Here's how the part is built. I have some questions about the finished solid (model axes, mm). Face numbers are marked on the shaded views. A direction names the side the tool comes from. Coordinates: 2 decimals unless noted, no trailing zeros. Write each loop counter-clockwise with the first axis right and the second up, starting at its lowest first coordinate (ties: lowest second). Pieces come first, ordered by that corner, then holes.
(1) Imagine slicing it at C-C, the plane z = -7. List the corners of the cut face in (x, y) for me, plus the area to 3 significant figures.
(2) Thinking about a two-plate mould opening in Z: for the marked faces 3 and 4, which applies, released by +Z, released by -Z, zero draft, split by the parting line, or undercut?
(3) Imagine slicing it at A-A, the plane z = 0. State how many separate pieces and enclosed holes the cut face has, plus the area to 3 significant figures.
(4) Imagine slicing it at D-D, the plane y = 5.75. List the corners of the cut face in (x, z) for me, plus the area to 3 significant figures.
(5) Please list where these lines run through material, in increasing order: probe 1 along X at (y, z) = (5.9, 0); probe 2 along Y at (x, z) = (16.5, 21.5); probe 3 along Z at (x, y) = (0, 8.4).
(6) Which directions (+Z, -Z, +X, -X, +Y, -Y) give clear straight access to the entire face, cutting with the end or side of a thin tool? Please do the marked faces 1 and 2.
(7) For pin 1 Ø5.5 at (x, z) = (-7, 0) entering from -Y; pin 2 Ø1.5 at (x, y) = (11, 1) entering from -Z; pin 3 Ø1 at (x, y) = (5, 6.5) entering from +Z, each with a flat end and sliding along its axis, tell me the tip position at first contact or that it passes through.
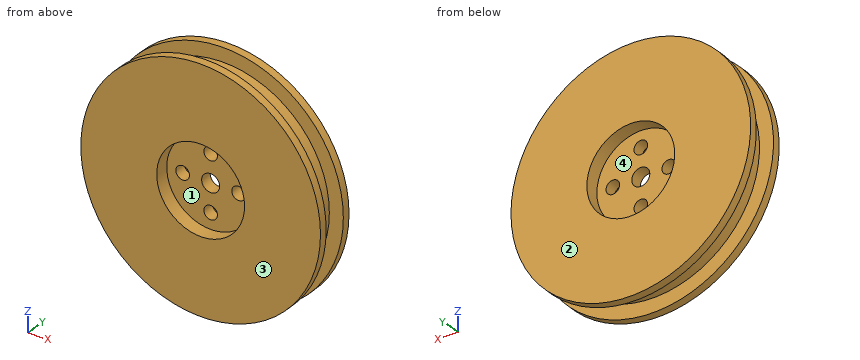
```python
from build123d import *

# Parameters (mm, degrees)
SKETCH1_R           = 30
EXTRUDE_C_DEPTH     = 2
SKETCH2_R           = 26.5
BOSS_EXTRUDE2_DEPTH = 6
SKETCH3_R           = 30
BOSS_EXTRUDE3_DEPTH = 2
SKETCH8_R           = 11
CUT_EXTRUDE2_DEPTH  = 3.5
SKETCH9_R           = 11
CUT_EXTRUDE3_DEPTH  = 3.5
SKETCH10_R          = 2.25
CUT_EXTRUDE4_DEPTH  = 12.5
SKETCH12_R          = 1.7
CUT_EXTRUDE5_DEPTH  = 10


with BuildPart() as part:
    # Sketch1 → Extrude c (new body)
    with BuildSketch(Plane(origin=(0, 0, 0), x_dir=(1, 0, 0), z_dir=(0, 1, 0))):
        Circle(SKETCH1_R)
    extrude(amount=EXTRUDE_C_DEPTH)

    # Sketch2 → Boss-Extrude2 (add)
    with BuildSketch(Plane(origin=(0, 2, 0), x_dir=(1, 0, 0), z_dir=(0, 1, 0))):
        Circle(SKETCH2_R)
    extrude(amount=BOSS_EXTRUDE2_DEPTH)

    # Sketch3 → Boss-Extrude3 (add)
    with BuildSketch(Plane(origin=(0, 8, 0), x_dir=(1, 0, 0), z_dir=(0, 1, 0))):
        Circle(SKETCH3_R)
    extrude(amount=BOSS_EXTRUDE3_DEPTH)

    # Sketch8 → Cut-Extrude2 (cut)
    with BuildSketch(Plane.XZ):
        Circle(SKETCH8_R)
    extrude(amount=-CUT_EXTRUDE2_DEPTH, mode=Mode.SUBTRACT)

    # Sketch9 → Cut-Extrude3 (cut)
    with BuildSketch(Plane(origin=(0, 10, 0), x_dir=(1, 0, 0), z_dir=(0, 1, 0))):
        Circle(SKETCH9_R)
    extrude(amount=-CUT_EXTRUDE3_DEPTH, mode=Mode.SUBTRACT)

    # Sketch10 → Cut-Extrude4 (cut)
    with BuildSketch(Plane(origin=(0, 6.5, 0), x_dir=(1, 0, 0), z_dir=(0, 1, 0))):
        Circle(SKETCH10_R)
    extrude(amount=-CUT_EXTRUDE4_DEPTH, mode=Mode.SUBTRACT)

    # Sketch12 → Cut-Extrude5 (cut)
    with BuildSketch(Plane(origin=(0, 6.5, 0), x_dir=(1, 0, 0), z_dir=(0, 1, 0))):
        with Locations((0, 7)):
            Circle(SKETCH12_R)
        with Locations((7, 0)):
            Circle(SKETCH12_R)
        with Locations((0, -7)):
            Circle(SKETCH12_R)
        with Locations((-7, 0)):
            Circle(SKETCH12_R)
    extrude(amount=-CUT_EXTRUDE5_DEPTH, mode=Mode.SUBTRACT)


solid = part.part
```
Recorded:
1. outline: (-29.17, 0) - (-8.49, 0) - (-8.49, 3.5) - (-1.7, 3.5) - (-1.7, 6.5) - (-8.49, 6.5) - (-8.49, 10) - (-29.17, 10) - (-29.17, 8) - (-25.56, 8) - (-25.56, 2) - (-29.17, 2) - close; (1.7, 3.5) - (8.49, 3.5) - (8.49, 0) - (29.17, 0) - (29.17, 2) - (25.56, 2) - (25.56, 8) - (29.17, 8) - (29.17, 10) - (8.49, 10) - (8.49, 6.5) - (1.7, 6.5) - close
1. area: 411 mm2
2. face 3: zero draft
2. face 4: undercut
3. separate pieces: 4
3. enclosed holes: 0
3. area: 370 mm2
4. outline: circle Ø53 at (0, 0); hole circle Ø3.4 at (-7, 0); hole circle Ø4.5 at (0, 0); hole circle Ø3.4 at (0, -7); hole circle Ø3.4 at (0, 7); hole circle Ø3.4 at (7, 0)
4. area: 2,150 mm2
5. probe 1: x = -26.5 to -8.7, -5.3 to -2.25, 2.25 to 5.3, 8.7 to 26.5
5. probe 2: y = 0 to 2, 8 to 10
5. probe 3: z = -30 to -11, 11 to 30
6. face 1: -Y
6. face 2: +Z, -Z, +X, -X, +Y
7. pin 1: stops at y = 3.5
7. pin 2: stops at z = -28.19
7. pin 3: stops at z = 26.12
